```python
from build123d import *

# Parameters (mm, degrees)
SKETCH1_R           = 3.5
BOSS_EXTRUDE1_DEPTH = 14
SKETCH2_W           = 7.5
SKETCH2_H           = 2
BOSS_EXTRUDE2_DEPTH = 14
CUT_EXTRUDE1_START  = -6.25
SKETCH4_R           = 3.5
SKETCH4_R_2         = 1.125
CUT_EXTRUDE1_DEPTH  = 6.25
SKETCH5_R           = 3.5
SKETCH5_R_2         = 1.125
CUT_EXTRUDE2_DEPTH  = 6.25
CUT_EXTRUDE3_DEPTH  = 17.507574019
SKETCH7_W           = 5
SKETCH7_H           = 5
BOSS_EXTRUDE3_DEPTH = 5
CUT_EXTRUDE4_DEPTH  = 19.506755523
CUT_EXTRUDE5_DEPTH  = 5
FILLET1_R           = 0.1
CUT_EXTRUDE6_DEPTH  = 5


with BuildPart() as part:
    # Sketch1 → Boss-Extrude1 (new body)
    with BuildSketch(Plane(origin=(0, 0, 0), x_dir=(0, 0, -1), z_dir=(1, 0, 0))):
        Circle(SKETCH1_R)
    extrude(amount=BOSS_EXTRUDE1_DEPTH)

    # Sketch2 → Boss-Extrude2 (add)
    with BuildSketch(Plane(origin=(0, 0, 0), x_dir=(0, 0, -1), z_dir=(1, 0, 0))):
        with Locations((0, 3.5)):
            Rectangle(SKETCH2_W, SKETCH2_H)
    extrude(amount=BOSS_EXTRUDE2_DEPTH)

    # Sketch4 → Cut-Extrude1 (cut)
    with BuildSketch(Plane(origin=(14, 0, 0), x_dir=(0, 0, -1), z_dir=(1, 0, 0)).offset(CUT_EXTRUDE1_START)):
        Circle(SKETCH4_R)
        Circle(SKETCH4_R_2, mode=Mode.SUBTRACT)
    extrude(amount=CUT_EXTRUDE1_DEPTH, mode=Mode.SUBTRACT)

    # Sketch5 → Cut-Extrude2 (cut)
    with BuildSketch(Plane.ZY):
        Circle(SKETCH5_R)
        with Locations(Location((0, 0, 0), (0, 0, 180))):
            Circle(SKETCH5_R_2, mode=Mode.SUBTRACT)
    extrude(amount=-CUT_EXTRUDE2_DEPTH, mode=Mode.SUBTRACT)

    # Sketch6 → Cut-Extrude3 (cut, through all)
    with BuildSketch(Plane.XY.offset(3.75)):
        Polygon((0, -1.495013081), (0, 1.709332254), (4.5, 1.709332254), (4.5, 0.875), (3.5, 0.875), (3.5, -1.495013081), align=None)
        Polygon((10.5, 0.875), (10.5, -1.495013081), (14, -1.495013081), (14, 1.709332254), (9.5, 1.709332254), (9.5, 0.875), align=None)
    extrude(amount=-CUT_EXTRUDE3_DEPTH, mode=Mode.SUBTRACT)

    # Sketch7 → Boss-Extrude3 (add)
    with BuildSketch(Plane(origin=(0, 4.5, 0), x_dir=(1, 0, 0), z_dir=(0, 1, 0))):
        with Locations((2.98, 0)):
            Rectangle(SKETCH7_W, SKETCH7_H)
        with Locations((11.02, 0)):
            Rectangle(SKETCH7_W, SKETCH7_H)
    extrude(amount=BOSS_EXTRUDE3_DEPTH)

    # Sketch8 → Cut-Extrude4 (cut, through all)
    with BuildSketch(Plane.XY.offset(3.75)):
        Polygon((2.157769387, 15.515103022), (0.48, 15.515103022), (0.48, 6), align=None)
        Polygon((13.52, 6), (11.842230613, 15.515103022), (13.52, 15.515103022), align=None)
    extrude(amount=-CUT_EXTRUDE4_DEPTH, mode=Mode.SUBTRACT)

    # Sketch9 → Cut-Extrude5 (cut)
    with BuildSketch(Plane(origin=(0, 9.5, 0), x_dir=(1, 0, 0), z_dir=(0, 1, 0))):
        with BuildLine():
            Line((4.48, 2.5), (5.48, 2.5))
            Line((5.48, 2.5), (5.48, 1.5))
            ThreePointArc((5.48, 1.5), (4.82498551, 1.84498551), (4.48, 2.5))
        make_face()
        with BuildLine():
            Line((0.48, 2.5), (0.48, 1.5))
            ThreePointArc((0.48, 1.5), (1.13501449, 1.84498551), (1.48, 2.5))
            Line((1.48, 2.5), (0.48, 2.5))
        make_face()
        with BuildLine():
            Line((5.48, -2.5), (5.48, -1.5))
            ThreePointArc((5.48, -1.5), (4.82498551, -1.84498551), (4.48, -2.5))
            Line((4.48, -2.5), (5.48, -2.5))
        make_face()
        with BuildLine():
            Line((0.48, -2.5), (0.48, -1.5))
            ThreePointArc((0.48, -1.5), (1.13501449, -1.84498551), (1.48, -2.5))
            Line((1.48, -2.5), (0.48, -2.5))
        make_face()
        with BuildLine():
            Line((8.52, -2.5), (8.52, -1.5))
            ThreePointArc((8.52, -1.5), (9.17501449, -1.84498551), (9.52, -2.5))
            Line((9.52, -2.5), (8.52, -2.5))
        make_face()
        with BuildLine():
            Line((12.52, -2.5), (13.52, -2.5))
            Line((13.52, -2.5), (13.52, -1.5))
            ThreePointArc((13.52, -1.5), (12.86498551, -1.84498551), (12.52, -2.5))
        make_face()
        with BuildLine():
            Line((13.52, 2.5), (13.52, 1.5))
            ThreePointArc((13.52, 1.5), (12.86498551, 1.84498551), (12.52, 2.5))
            Line((12.52, 2.5), (13.52, 2.5))
        make_face()
        with BuildLine():
            Line((8.52, 2.5), (8.52, 1.5))
            ThreePointArc((8.52, 1.5), (9.17501449, 1.84498551), (9.52, 2.5))
            Line((9.52, 2.5), (8.52, 2.5))
        make_face()
    extrude(amount=-CUT_EXTRUDE5_DEPTH, mode=Mode.SUBTRACT)

    # Fillet1
    fillet1_edges = [part.edges().sort_by_distance(p)[0] for p in [
        (1.097144432, 9.5, 0),
        (2.98, 9.5, -2.5),
        (4.82498551, 9.5, -1.84498551),
        (5.48, 9.5, 0),
        (4.82498551, 9.5, 1.84498551),
        (2.98, 9.5, 2.5),
        (8.52, 9.5, 0),
        (9.17501449, 9.5, -1.84498551),
        (11.02, 9.5, -2.5),
        (12.902855568, 9.5, 0),
        (11.02, 9.5, 2.5),
        (9.17501449, 9.5, 1.84498551),
        (1.344642616, 9.5, -2.123284662),
        (1.344642616, 9.5, 2.123284662),
        (12.655357384, 9.5, -2.123284662),
        (12.655357384, 9.5, 2.123284662),
    ]]
    fillet(fillet1_edges, radius=FILLET1_R)

    # Sketch10 → Cut-Extrude6 (cut)
    with BuildSketch(Plane(origin=(0, 9.5, 0), x_dir=(1, 0, 0), z_dir=(0, 1, 0))):
        with BuildLine():
            Line((1.48, 1.25), (1.48, -1.25))
            ThreePointArc((1.48, -1.25), (4.932562419, 0), (1.48, 1.25))
        make_face()
        with BuildLine():
            Line((12.52, 1.25), (12.52, -1.25))
            ThreePointArc((12.52, -1.25), (9.067437581, 0), (12.52, 1.25))
        make_face()
    extrude(amount=-CUT_EXTRUDE6_DEPTH, mode=Mode.SUBTRACT)


solid = part.part
```
Check sheet for the modelled part. Datum: model origin and axes. Units: mm. A direction names the side the tool comes from. Coordinates: 2 decimals unless noted, no trailing zeros. Order: outer loops, then holes, each group sorted by start corner. A loop starts at its lowest first (then second) coordinate and runs counter-clockwise, first axis right, second up. Notation, with made-up numbers: (89, 89.25) -> (117, 89.25) arc R3 ccw to (117, 93.25) -> close; hole circle Ø10 at (88.25, -17). An arc over 180 degrees is marked (long way). Write item = value, one per line. Start each with the question number.
1) Mould release check, pull along Y, two halves, no side actions. Record for faces 6 (the cylindrical face through (7, -3.5, 0.1)), 7 (the flat face through (7, 4.5, 0)), 8 (the cylindrical face through (4.856, -1.115, 0.146)), 9 (the flat face through (3, 7, -2.5)): +Y half, -Y half, draft (parallel to the pull), parting line (faces both ways), or undercut.
2) Cross-section at C-C (x = 2.98). Enter the section's corners in (y, z).
3) Cross-section at A-A (x = 8). Enter the section's corners in (y, z) (3 decimals).
4) Cross-section at D-D (y = 0). Enter the section's corners in (x, z) (3 decimals), then the cut area to 3 significant figures.
5) Material ranges on L1, parallel to X at y = 7.25, z = -0.5; L2, parallel to Z at x = 2.98, y = 8.4; L3, parallel to X at y = 6.5, z = -0.5, recorded low to high.
6) Go/stop test with flat-tipped pins: P1, Ø1.5, axis at x = 11, y = 8, coming from the -Z side; P2, Ø2, axis at x = 9.5, z = 1, coming from the -Y side (3 decimals); P3, Ø2.5, axis at x = 11, y = 6, coming from the +Z side; P4, Ø1, axis at x = 6.5, y = 6.5, coming from the -Z side. Record where each tip stops, or that it passes through.
7) Access from +Z, -Z, +X, -X, +Y, -Y to the whole of each face (thin tool, end or side, straight path). Record for faces 1 (the cylindrical face through (4.83, 6.98, 1.84)), 2 (the flat face through (4, 0.875, 0)), 3 (the cylindrical face through (9.07, 7.04, 0.07)), 4 (the cylindrical face through (12.762, 6.984, 1.962)), 5 (the flat face through (10, 0.875, 0)).
8) Cross-section at B-B (y = 6.5). Enter the section's corners in (x, z), then the cut area to 3 significant figures.
Ans:
q1.face_6 = undercut
q1.face_7 = +Y half
q1.face_8 = undercut
q1.face_9 = draft
q2.outline = (2.5, -3.75) -> (4.5, -3.75) -> (4.5, -2.5) -> (9.4, -2.5) arc R0.1 ccw to (9.5, -2.4) -> (9.5, -1.95) -> (4.5, -1.95) -> (4.5, 1.95) -> (9.5, 1.95) -> (9.5, 2.4) arc R0.1 ccw to (9.4, 2.5) -> (4.5, 2.5) -> (4.5, 3.75) -> (2.5, 3.75) -> (2.5, 2.45) arc R3.5 cw to (2.5, -2.45) -> close
q3.outline = circle Ø2.25 at (0, 0); (2.5, -3.75) -> (4.5, -3.75) -> (4.5, 3.75) -> (2.5, 3.75) -> (2.5, 2.449) arc R3.5 cw to (2.5, -2.449) -> close
q4.outline = (3.5, -1.125) -> (6.25, -1.125) -> (6.25, -3.5) -> (7.75, -3.5) -> (7.75, -1.125) -> (10.5, -1.125) -> (10.5, 1.125) -> (7.75, 1.125) -> (7.75, 3.5) -> (6.25, 3.5) -> (6.25, 1.125) -> (3.5, 1.125) -> close
q4.area = 22.9 mm²
q5.L1 = 0.7 to 1.48, 4.87 to 5.48, 8.52 to 9.13, 12.52 to 13.3
q5.L2 = -2.5 to -1.95, 1.95 to 2.5
q5.L3 = 0.57 to 1.48, 4.87 to 5.48, 8.52 to 9.13, 12.52 to 13.43
q6.P1 = -2.5
q6.P2 = -1.125
q6.P3 = 2.5
q6.P4 = through
q7.face_1 = +Z, +Y
q7.face_2 = +Z, -Z, -X
q7.face_3 = +Y
q7.face_4 = +Z, +X, +Y
q7.face_5 = +Z, -Z, +X
q8.outline = (0.57, -1.52) arc R1.25 cw to (1.48, -2.5) -> (4.48, -2.5) arc R1.25 cw to (5.48, -1.5) -> (5.48, 1.5) arc R1.25 cw to (4.48, 2.5) -> (1.48, 2.5) arc R1.25 cw to (0.57, 1.52) -> close; (8.52, -1.5) arc R1.25 cw to (9.52, -2.5) -> (12.52, -2.5) arc R1.25 cw to (13.43, -1.52) -> (13.43, 1.52) arc R1.25 cw to (12.52, 2.5) -> (9.52, 2.5) arc R1.25 cw to (8.52, 1.5) -> close; hole (1.48, -1.25) arc R1.95 ccw (long way) to (1.48, 1.25) -> close; hole (12.52, -1.25) -> (12.52, 1.25) arc R1.95 ccw (long way) to start
q8.area = 21.4 mm²
